Work out the finished part from the listing and answer in its coordinate system (mm). A direction names the side the tool comes from. Round coordinates to 2 decimals unless told otherwise and drop trailing zeros. Loops run counter-clockwise (first coordinate to the right, second up) from the corner with the lowest first, then second, coordinate; pieces in that order, holes last. Notation, with made-up numbers: (6, -10.75) - (49, -10.75) arc R13 ccw to (49, 0.25) - close; hole circle Ø7 at (85, -28.5). An arc over 180 degrees is marked (long way). Return JSON: item names as keys, results as strings.
Autodesk Inventor part; units mm, degrees
ref_plane "Work Plane3" through (0, 5, 0) normal (0, 1, 0) x (1, 0, 0)
ref_plane "YZ Plane" through (0, 0, 0) normal (1, 0, 0) x (0, 1, 0)
ref_plane "XZ Plane" through (0, 0, 0) normal (0, 1, 0) x (-1, 0, 0)
sketch "Sketch1" plane through (0, 0, 0) normal (0, 1, 0) x (-1, 0, 0)
  line L0 (30, 30) -> (-30, 30)
  line L1 (-30, 30) -> (-30, -30)
  line L2 (-30, -30) -> (30, -30)
  line L3 (30, -30) -> (30, 30)
  line L4 (30, 30) -> (-30, -30) construction
  line L5 (-30, 30) -> (30, -30) construction
  point P0 (0, 0)
  dimension "d0" = 60
  dimension "d1" = 60
extrude "Extrusion1" add sketch "Sketch1" along normal blind 10
fillet "Fillet1" radius 7 4 edges at (30, 5, 30) (30, 5, -30) (-30, 5, 30) (-30, 5, -30)
sketch "Sketch2" plane through (0, 10, 0) normal (0, 1, 0) x (1, 0, 0)
  line L0 (-30, 30) -> (30, 30)
  line L1 (30, 30) -> (30, -30)
  line L2 (30, -30) -> (-30, -30)
  line L3 (-30, -30) -> (-30, 30)
  line L4 (-30, 30) -> (30, -30) construction
  line L5 (30, 30) -> (-30, -30) construction
  line L6 (25, -25) -> (25, 25)
  line L7 (25, 25) -> (-25, 25)
  line L8 (-25, 25) -> (-25, -25)
  line L9 (-25, -25) -> (25, -25)
  circle A0 centre (25, -25) radius 2.75
  circle A1 centre (-25, -25) radius 2.75
  circle A2 centre (25, 25) radius 2.75
  circle A3 centre (-25, 25) radius 2.75
  point P0 (0, 0)
  dimension "d5" = 5
  dimension "d6" = 5.5
  dimension "d7" = 5.5
  dimension "d8" = 5.5
  dimension "d9" = 5.5
extrude "Extrusion2" cut sketch "Sketch2" against normal blind 3 contours L9 A0 L6 | L6 A0 L9 | A2 L7 L6 | L6 L7 A2 | A1 L8 L9 | L9 L8 A1 | A3 L8 L7 | L7 L8 A3
sketch "Sketch7" plane through (0, 10, 0) normal (0, 1, 0) x (1, 0, 0)
  line L0 (-23, 30) -> (23, 30)
  line L1 (30, 23) -> (30, -23)
  line L2 (23, -30) -> (-23, -30)
  line L3 (-30, -23) -> (-30, 23)
  line L4 (-30, 30) -> (30, -30) construction
  line L5 (30, 30) -> (-30, -30) construction
  arc A0 (-23, 30) -> (-30, 23) centre (-23, 23) ccw
  arc A1 (-30, -23) -> (-23, -30) centre (-23, -23) ccw
  arc A2 (23, -30) -> (30, -23) centre (23, -23) ccw
  arc A3 (30, 23) -> (23, 30) centre (23, 23) ccw
  line L6 (23, 32) -> (-23, 32)
  arc A4 (-23, 32) -> (-32, 23) centre (-23, 23) ccw
  line L7 (-32, 23) -> (-32, -23)
  arc A5 (-32, -23) -> (-23, -32) centre (-23, -23) ccw
  line L8 (-23, -32) -> (23, -32)
  arc A6 (23, -32) -> (32, -23) centre (23, -23) ccw
  line L9 (32, -23) -> (32, 23)
  arc A7 (32, 23) -> (23, 32) centre (23, 23) ccw
  point P0 (0, 0)
  dimension "d47" = 7
  dimension "d48" = 2
extrude "Extrusion6" add sketch "Sketch7" against normal blind 10
sketch "Sketch14" plane through (0, 10, 0) normal (0, 1, 0) x (1, 0, 0)
  line L0 (-25, 25) -> (25, 25)
  line L1 (25, 25) -> (25, -25)
  line L2 (25, -25) -> (-25, -25)
  line L3 (-25, -25) -> (-25, 25)
  line L4 (-25, 25) -> (25, -25) construction
  line L5 (25, 25) -> (-25, -25) construction
  line L6 (21, -21) -> (21, 2.7)
  line L7 (21, 21) -> (-21, 21)
  line L8 (-21, 21) -> (-21, -21)
  line L9 (-16.3, -21) -> (21, -21)
  line L10 (-16.3, -21) -> (-16.3, 2.7)
  line L11 (21, 2.7) -> (-16.3, 2.7)
  line L12 (19, 0.7) -> (-14.3, 0.7)
  line L13 (-14.3, 0.7) -> (-14.3, -19)
  line L14 (-19, -19) -> (-19, 19)
  line L15 (-19, 19) -> (19, 19)
  line L16 (19, -19) -> (-14.3, -19)
  line L17 (19, 0.7) -> (19, -19)
  point P0 (0, 0)
  dimension "d95" = 50
  dimension "d96" = 50
  dimension "d97" = 4
  dimension "d98" = 37.3
  dimension "d99" = 23.7
  dimension "d100" = 2
extrude "Extrusion12" cut sketch "Sketch14" against normal blind 2 contours L9 L10 L11 L6
sketch "Sketch15" plane through (0, 10, 0) normal (0, 1, 0) x (1, 0, 0)
  line L0 (-14.3, 0.7) -> (19, 0.7)
  line L1 (19, 0.7) -> (19, -19)
  line L2 (19, -19) -> (-14.3, -19)
  line L3 (-14.3, -19) -> (-14.3, 0.7)
  point P0 (0, 0)
extrude "Extrusion13" cut sketch "Sketch15" against normal blind 8
sketch "Sketch16" plane through (0, 10, 0) normal (0, 1, 0) x (1, 0, 0)
  line L0 (23, 32) -> (-23, 32)
  line L1 (-32, 23) -> (-32, -23)
  line L2 (32, -23) -> (32, 23)
  line L3 (-18, 28) -> (18, 28)
  line L4 (-16.3, 2.7) -> (21, 2.7)
  line L5 (-18, 28) -> (-18, 6.7)
  line L6 (-18, 6.7) -> (18, 6.7)
  line L7 (18, 18) -> (18, 28)
  line L8 (-23, -32) -> (23, -32)
  line L9 (-16.3, -21) -> (-16.3, 2.7)
  line L10 (-28, -18) -> (-20.3, -18)
  line L11 (-20.3, -18) -> (-20.3, 2.7)
  line L12 (-28, -18) -> (-28, 18)
  line L13 (-20.3, 2.7) -> (-22, 2.7)
  line L14 (-22, 2.7) -> (-22, 6.7)
  line L15 (-28, 18) -> (-22, 18)
  line L16 (-22, 18) -> (-22, 6.7)
  line L17 (21, -21) -> (-16.3, -21)
  line L18 (18, -28) -> (18, -25)
  line L19 (18, -25) -> (-18, -25)
  line L20 (18, -28) -> (-18, -28)
  line L21 (-18, -28) -> (-18, -25)
  line L22 (21, 2.7) -> (21, -21)
  line L23 (28, 18) -> (28, -18)
  line L24 (28, -18) -> (25, -18)
  line L25 (25, -18) -> (25, 18)
  line L26 (28, 18) -> (25, 18)
  line L27 (21, 18) -> (21, 6.7)
  line L28 (21, 6.7) -> (18, 6.7)
  line L29 (21, 18) -> (18, 18)
  point P0 (0, 0)
  dimension "d106" = 4
  dimension "d107" = 4
  dimension "d108" = 14
  dimension "d109" = 14
  dimension "d110" = 4
  dimension "d111" = 4
  dimension "d112" = 4
  dimension "d113" = 14
  dimension "d114" = 4
  dimension "d115" = 14
  dimension "d116" = 4
  dimension "d117" = 4
  dimension "d118" = 4
  dimension "d119" = 4
  dimension "d120" = 4
  dimension "d121" = 14
  dimension "d122" = 4
  dimension "d123" = 14
  dimension "d124" = 4
  dimension "d125" = 14
  dimension "d126" = 4
  dimension "d127" = 4
  dimension "d128" = 14
  dimension "d129" = 4
extrude "Extrusion14" cut sketch "Sketch16" against normal through all contours L3 L7 L29 L27 L28 L6 L5 | L12 L15 L16 L14 L13 L11 L10 | L20 L21 L19 L18 | L23 L24 L25 L26
fillet "Fillet4" radius 2 8 edges at (18, 5, -28) (-22, 5, -18) (-18, 5, -28) (-28, 5, -18) (-28, 5, 18) (-18, 5, -6.7) (-20.3, 5, 18) (21, 5, -6.7)
fillet "Fillet4" radius 0.5 16 edges at (28, 5, 18) (18, 5, 28) (28, 5, -18) (21, 5, -18) (18, 5, -18) (18, 5, 25) (-20.3, 5, -2.7) (-22, 5, -2.7) (25, 5, -18) (-18, 5, 25) (-18, 5, 28) (25, 5, 18) (-14.3, 2, 9.15) (2.35, 2, -0.7) (2.35, 2, 19) (19, 2, 9.15)
ref_plane "Work Plane3" through (0, 5, 0) normal (0, 1, 0) x (1, 0, 0)
mirror "Mirror3" about plane through (0, 5, 0) normal (0, 1, 0) of "Extrusion2"
properties part number "14 pin short holder"
1) Section A-A (z = 4) is taken. Give the vertices of the cut face in (x, y), and give its area (3 significant figures).
Verdict:
{"outline": "(-32, 0) - (-28, 0) - (-28, 10) - (-32, 10) - close; (-20.3, 0) - (25, 0) - (25, 10) - (21, 10) - (21, 8) - (19, 8) - (19, 2.5) arc R0.5 cw to (18.5, 2) - (-13.8, 2) arc R0.5 cw to (-14.3, 2.5) - (-14.3, 8) - (-16.3, 8) - (-16.3, 10) - (-20.3, 10) - close; (28, 0) - (32, 0) - (32, 10) - (28, 10) - close", "area": "259 mm2"}
2) Section B-B (x = -25) is taken. Give the vertices of the cut face in (y, z).
Verdict:
{"outline": "(0, -31.77) - (10, -31.77) - (10, -27.75) - (7, -27.75) - (7, -22.25) - (10, -22.25) - (10, -18) - (0, -18) - (0, -22.25) - (3, -22.25) - (3, -27.75) - (0, -27.75) - close; (0, 18) - (10, 18) - (10, 22.25) - (7, 22.25) - (7, 27.75) - (10, 27.75) - (10, 31.77) - (0, 31.77) - (0, 27.75) - (3, 27.75) - (3, 22.25) - (0, 22.25) - close"}
3) Section D-D (z = -13) is taken. Give the vertices of the cut face in (x, y).
Verdict:
{"outline": "(-32, 0) - (-28, 0) - (-28, 10) - (-32, 10) - close; (-22, 0) - (-18, 0) - (-18, 10) - (-22, 10) - close; (21, 0) - (25, 0) - (25, 10) - (21, 10) - close; (28, 0) - (32, 0) - (32, 10) - (28, 10) - close"}
4) A tool of negligible diameter and unlimited length cuts with its end or side. For faces 1 (the flat face through (-25, 7, -25)), 2 (the cylindrical face through (-27.43, 4.93, -17.4)), 3 (the cylindrical face through (-27.747, 1.479, -24.879)), from which of +Z, -Z, +X, -X, +Y, -Y can it reach the whole face along a straight path? Write none if from no direction.
Verdict:
{"face 1": "+Y", "face 2": "+Y, -Y", "face 3": "-Y"}
5) Section C-C (x = -13) is taken. Give the vertices of the cut face in (y, z).
Verdict:
{"outline": "(0, -32) - (10, -32) - (10, -28) - (0, -28) - close; (0, -6.7) - (10, -6.7) - (10, -2.7) - (8, -2.7) - (8, -0.7) - (2.5, -0.7) arc R0.5 cw to (2, -0.2) - (2, 18.5) arc R0.5 cw to (2.5, 19) - (8, 19) - (8, 21) - (10, 21) - (10, 25) - (0, 25) - close; (0, 28) - (10, 28) - (10, 32) - (0, 32) - close"}
6) Find the intervals of material crossed by L1, parallel to X at y = 3.5, z = 6; L2, parallel to X at y = 1.25, z = -6; L3, parallel to Z at x = -8.5, y = 2.75, in increasing order.
Verdict:
{"L1": "x = -32 to -28, -20.3 to -14.3, 19 to 25, 28 to 32", "L2": "x = -32 to -28, -22 to 25, 28 to 32", "L3": "z = -32 to -28, -6.7 to -0.7, 19 to 25, 28 to 32"}
7) Determine the mould class of faces 4 (the flat face through (-18, 5, -17)), 5 (the flat face through (0, 5, 32)), 6 (the flat face through (-32, 5, 0)) for opening direction X: pulls with the +X half, pulls with the -X half, needs draft (parallel to the pull), parting line crosses it, or undercut.
Verdict:
{"face 4": "undercut", "face 5": "needs draft", "face 6": "pulls with the -X half"}
8) Flat-ended cylindrical pins translate along their axes: pin 1 (1 mm diameter, centred on x = 26.5, y = 5, fed in from -Z); pin 2 (5 mm diameter, centred on x = 25, z = 25, fed in from -Y); pin 3 (4.5 mm diameter, centred on x = -25, z = 25, fed in from +Y). Find the tip coordinate at first contact, or state that the pin passes through.
Verdict:
{"pin 1": "stops at z = -31.49", "pin 2": "stops at y = 3", "pin 3": "stops at y = 7"}
